from build123d import *

# Parameters (mm, degrees)
EXTRUSION1_DEPTH        = 0.8
ESQUISSE2_R             = 0.89
ENL_V_MAT_EXTRU_1_DEPTH = 0.8
CHANFREIN1_SIZE         = 0.4
CHANFREIN2_SIZE         = 0.4


with BuildPart() as part:
    # Esquisse1 → Extrusion1 (new body)
    with BuildSketch(Plane(origin=(0, 0, 0), x_dir=(0, 1, 0), z_dir=(0, 0, 1))):
        Polygon((-3.96, 0.034), (-3.08, 0.034), (-3.08, -2.791082591), (-1.94, -2.791082591), (-1.94, 0.034), (1.94, 0.034), (1.94, -2.791082591), (3.08, -2.791082591), (3.08, 0.034), (3.96, 0.034), (3.96, 2.484), (3.11, 2.484), (3.11, 15.553159959), (2.464351087, 16.2), (-2.464351087, 16.2), (-3.11, 15.553159959), (-3.11, 2.484), (-3.96, 2.484), align=None)
    extrude(amount=EXTRUSION1_DEPTH)

    # Esquisse2 → Enlèv. mat.-Extru.1 (cut)
    with BuildSketch(Plane(origin=(0, 0, 0.8), x_dir=(0, 1, 0), z_dir=(0, 0, 1))):
        with Locations(Location((0, 11.68, 0), (0, 0, 180))):
            Circle(ESQUISSE2_R)
    extrude(amount=-ENL_V_MAT_EXTRU_1_DEPTH, mode=Mode.SUBTRACT)

    # Chanfrein1
    chanfrein1_edges = [part.edges().sort_by_distance(p)[0] for p in [
        (-16.2, 0, 0),
    ]]
    chamfer(chanfrein1_edges, length=CHANFREIN1_SIZE)

    # Chanfrein2
    chanfrein2_edges = [part.edges().sort_by_distance(p)[0] for p in [
        (-16.2, 0, 0.8),
    ]]
    chamfer(chanfrein2_edges, length=CHANFREIN2_SIZE - 0.0001)  # a hair under: the kernel refuses the full size


solid = part.part
Verification items for the finished model (mm, model axes). Coordinates: 2 decimals unless noted, no trailing zeros. Order: outer loops, then holes, each group sorted by start corner. A loop starts at its lowest first (then second) coordinate and runs counter-clockwise, first axis right, second up. Notation, with made-up numbers: (69.25, -13.5) -> (114.25, -13.5) arc R16 cw to (114.25, 5.5) -> close; hole circle Ø6 at (-21, -39). An arc over 180 degrees is marked (long way). Use CSV: the item, a comma, the result in double quotes. Start each with the question number.
Q1. Section check C-C, the plane x = 1.5. Record the cut outline in (y, z).
Q2. Draft check along X on faces 1 (the cylindrical face through (-10.8, 0.12, 0.41)), 2 (the flat face through (-7, 0, 0.8)). Enter one of: +X half, -X half, draft (parallel to the pull), parting line (faces both ways), or undercut.
Q3. Section check A-A, the plane x = -11.68. Record the cut outline in (y, z).
Q4. Thickness scan on line 1 along Y through (x, z) = (1.5, 0.5); line 2 along Y through (x, z) = (-11.75, 0.6); line 3 along Y through (x, z) = (-10.25, 0.4). Record the ranges inside material, lowest first.
Q5. Depth check by flat-ended pin: P1, Ø2, axis at x = -12.5, y = 2.5, coming from the -Z side. Enter the tip coordinate at first touch or a pass-through.
Returned:
1,outline,"(-3.08, 0) -> (-1.94, 0) -> (-1.94, 0.8) -> (-3.08, 0.8) -> close; (1.94, 0) -> (3.08, 0) -> (3.08, 0.8) -> (1.94, 0.8) -> close"
2,face 1,"undercut"
2,face 2,"draft"
3,outline,"(-3.11, 0) -> (-0.89, 0) -> (-0.89, 0.8) -> (-3.11, 0.8) -> close; (0.89, 0) -> (3.11, 0) -> (3.11, 0.8) -> (0.89, 0.8) -> close"
4,line 1,"y = -3.08 to -1.94, 1.94 to 3.08"
4,line 2,"y = -3.11 to -0.89, 0.89 to 3.11"
4,line 3,"y = -3.11 to 3.11"
5,P1,"stops at z = 0"
